```python
from build123d import *

# Parameters (mm, degrees)
SKETCH1_R           = 25.48
BOSS_EXTRUDE1_DEPTH = 6
SKETCH10_R          = 2
BOSS_EXTRUDE3_DEPTH = 2


with BuildPart() as part:
    # Sketch1 → Boss-Extrude1 (new body)
    with BuildSketch(Plane.XY):
        Circle(SKETCH1_R)
    extrude(amount=BOSS_EXTRUDE1_DEPTH)

    # Sketch10 → Boss-Extrude3 (add)
    with BuildSketch(Plane(origin=(0, 0, 0), x_dir=(-1, 0, 0), z_dir=(0, 0, -1))):
        with Locations((0, 13.421433997)):
            Circle(SKETCH10_R)
        with Locations((11.623302797, 6.710716999)):
            Circle(SKETCH10_R)
        with Locations((11.623302797, -6.710716999)):
            Circle(SKETCH10_R)
        with Locations((0, -13.421433997)):
            Circle(SKETCH10_R)
        with Locations((-11.623302797, -6.710716999)):
            Circle(SKETCH10_R)
        with Locations((-11.623302797, 6.710716999)):
            Circle(SKETCH10_R)
    extrude(amount=BOSS_EXTRUDE3_DEPTH)


solid = part.part
```
CAD build for the part. Positions are in the model's coordinates, mm. A direction names the side the tool comes from. Coordinates: 2 decimals unless noted, no trailing zeros. Write each loop counter-clockwise with the first axis right and the second up, starting at its lowest first coordinate (ties: lowest second). Pieces come first, ordered by that corner, then holes.
(1) Cut at B-B, the plane z = 3.25. List the corners of the cut face in (x, y), and give its area (3 significant figures).
(2) 3-axis set-ups, long thin cutter, end or side, ignore diameter. For faces 1 (the face through (0, 0, 6)), 2 (the face through (9.776, 5.945, -0.986)): which of +Z, -Z, +X, -X, +Y, -Y reach the whole face in a straight line?
(3) Two-plate mould, pull along X, no slides. Class faces 3 (the face through (-0.923, -15.196, -0.986)), 4 (the face through (9.776, -7.477, -0.986)), 5 (the face through (12, -7, -2)): +X half, -X half, draft (parallel to the pull), parting line (faces both ways), or undercut.
(4) Cut at D-D, the plane x = -16.5. List the corners of the cut face in (y, z).
(5) Cut at C-C, the plane y = -19. List the corners of the cut face in (x, z), and give its area (3 significant figures).
(6) Cut at A-A, the plane x = 0. List the corners of the cut face in (y, z), and give its area (3 significant figures).
(7) Flat gauge pins, fed straight in: pin 1 (4 mm diameter, centred on y = 3.5, z = 2.5, fed in from +X); pin 2 (1.5 mm diameter, centred on x = 12.5, z = 1, fed in from +Y); pin 3 (1.5 mm diameter, centred on y = 16.5, z = -0.5, fed in from +X); pin 4 (12 mm diameter, centred on x = 16.5, y = 8.5, fed in from -Z). Where does each tip first touch, or does it go through?
(8) Drill centre lines: probe 1 along Z at (x, y) = (-0.5, -1); probe 2 along X at (y, z) = (-13, 1.25); probe 3 along X at (y, z) = (-8, 3.75). Where is each one in solid material? Low to high.
Geometry says:
1. outline: circle Ø50.96 at (0, 0)
1. area: 2,040 mm2
2. face 1: +Z, +X, -X, +Y, -Y
2. face 2: -Z
3. face 3: parting line
3. face 4: undercut
3. face 5: draft
4. outline: (-19.42, 0) - (19.42, 0) - (19.42, 6) - (-19.42, 6) - close
5. outline: (-16.98, 0) - (16.98, 0) - (16.98, 6) - (-16.98, 6) - close
5. area: 204 mm2
6. outline: (-25.48, 0) - (-15.42, 0) - (-15.42, -2) - (-11.42, -2) - (-11.42, 0) - (11.42, 0) - (11.42, -2) - (15.42, -2) - (15.42, 0) - (25.48, 0) - (25.48, 6) - (-25.48, 6) - close
6. area: 322 mm2
7. pin 1: stops at x = 25.44
7. pin 2: stops at y = 22.61
7. pin 3: stops at x = 19.88
7. pin 4: stops at z = -2
8. probe 1: z = 0 to 6
8. probe 2: x = -21.91 to 21.91
8. probe 3: x = -24.19 to 24.19
